Drawing for the job (mm, zero at the part's lowest x, y, z). Give positions to 0.01 mm unless a question says otherwise; leave off trailing zeros. Write each loop counter-clockwise with the first axis right and the second up, starting at its lowest first coordinate (ties: lowest second). Pieces come first, ordered by that corner, then holes.
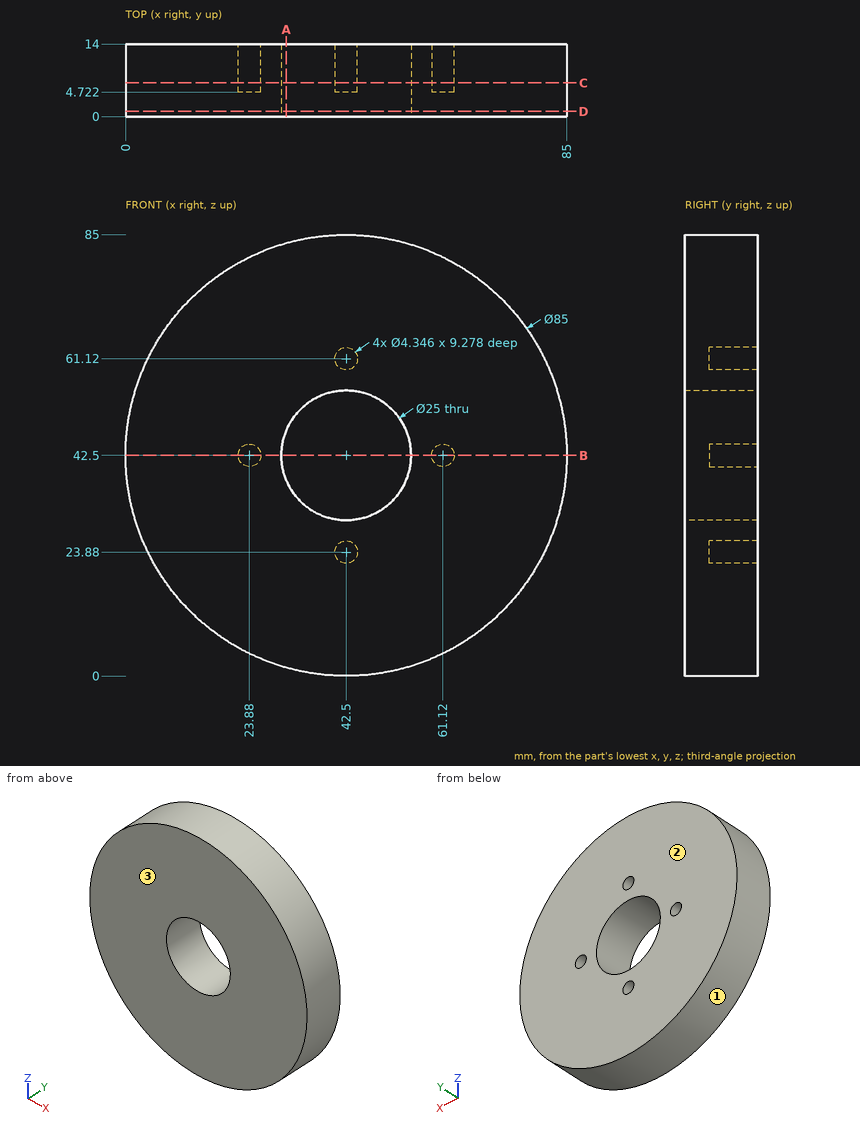
1. Slice it at B-B, the plane z = 42.5. Write the cut outline in (x, y).
Calculated:
outline: (0, 0) - (30, 0) - (30, 14) - (26.05, 14) - (26.05, 4.72) - (21.71, 4.72) - (21.71, 14) - (0, 14) - close; (55, 0) - (85, 0) - (85, 14) - (63.29, 14) - (63.29, 4.72) - (58.95, 4.72) - (58.95, 14) - (55, 14) - close
2. Slice it at C-C, the plane y = 6.5. Write the cut outline in (x, z).
Calculated:
outline: circle Ø85 at (42.5, 42.5); hole circle Ø4.35 at (23.88, 42.5); hole circle Ø25 at (42.5, 42.5); hole circle Ø4.35 at (42.5, 23.88); hole circle Ø4.35 at (42.5, 61.12); hole circle Ø4.35 at (61.12, 42.5)
3. Slice it at D-D, the plane y = 1. Write the cut outline in (x, z), and give its area (3 significant figures).
Calculated:
outline: circle Ø85 at (42.5, 42.5); hole circle Ø25 at (42.5, 42.5)
area: 5,180 mm2
4. Slice it at A-A, the plane x = 31. Write the cut outline in (y, z) (1 decimal).
Calculated:
outline: (0, 1.6) - (14, 1.6) - (14, 37.6) - (0, 37.6) - close; (0, 47.4) - (14, 47.4) - (14, 83.4) - (0, 83.4) - close
5. Pin check, flat tips, straight feed: P1, Ø4, axis at x = 42.5, z = 23.88, coming from the +Y side; P2, Ø4, axis at y = 6, z = 23.5, coming from the -X side; P3, Ø5, axis at y = 12, z = 11.5, coming from the +X side. Stop position of each tip, or through.
Calculated:
P1: stops at y = 4.72
P2: stops at x = 3.55
P3: stops at x = 74.03
6. Pull direction Y, two halves, no side cores. Call the marked faces 1, 2 and 3: +Y half, -Y half, draft (parallel to the pull), parting line (faces both ways), or undercut.
Calculated:
face 1: draft
face 2: +Y half
face 3: -Y half
7. Probe probe 1 along Z at (x, y) = (24, 10.75); probe 2 along Z at (x, y) = (34.5, 10.5) (1 decimal); probe 3 along X at (y, z) = (3.5, 42.5). List the from-to ranges inside material, lowest first.
Calculated:
probe 1: z = 4.24 to 40.33, 44.67 to 80.76
probe 2: z = 0.8 to 32.9, 52.1 to 84.2
probe 3: x = 0 to 30, 55 to 85
